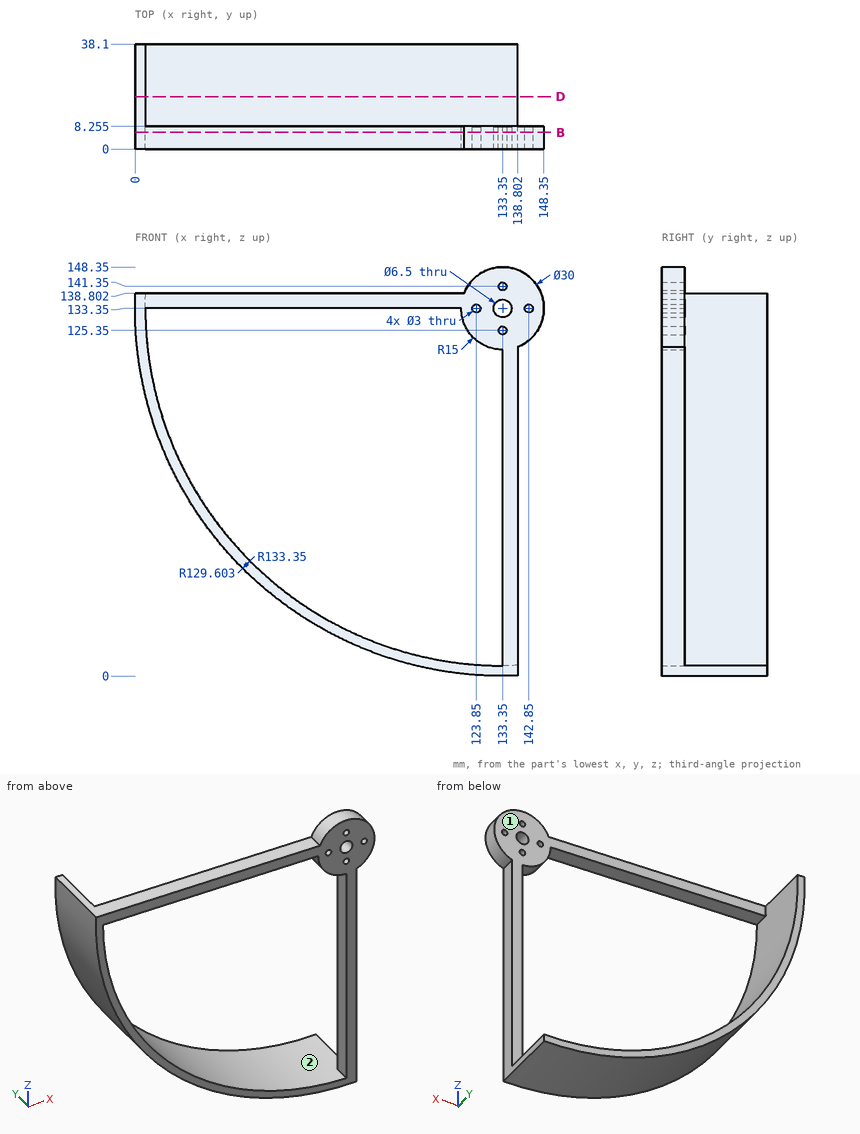
Here's the drawing with two shaded views (mm, measured from the low corner). I have some questions. Coordinates: 2 decimals unless noted, no trailing zeros. Write each loop counter-clockwise with the first axis right and the second up, starting at its lowest first coordinate (ties: lowest second). Pieces come first, ordered by that corner, then holes.
Item 1: I want a section at D-D on y = 19. Write out the boundary of the cut face in (x, z).
Item 2: If I drill on line 1 (Z direction, x = 123, y = 4) (1 decimal); line 2 (Z direction, x = 135, y = 6); line 3 (X direction, y = 5, z = 141.35), over which ranges is the centre line in solid material (lowest first)?
Item 3: I want a section at B-B on y = 6. Count the separate pieces of the cut face and the enclosed holes in it, and give its area (3 significant figures).
Item 4: Will these pins go through, and if not, where does the flat tip stop? pin 1 (19 mm diameter, centred on x = 66.5, y = 22, fed in from +Z); pin 2 (4 mm diameter, centred on x = 49, y = 6, fed in from -Z) (1 decimal); pin 3 (3 mm diameter, centred on y = 22, z = 68, fed in from -X); pin 4 (10.5 mm diameter, centred on x = 133.35, z = 133.35, fed in from -Y).
Item 5: If we mould it in two halves opening along Z, with no side actions, what happens to the marked faces 1 and 2? For each: +Z half, -Z half, draft (parallel to the pull), parting line (faces both ways), or undercut.
Findings below:
1. outline: (0.11, 138.8) arc R133.35 ccw to (138.8, 0.11) - (138.8, 3.86) arc R129.6 cw to (3.86, 138.8) - close
2. line 1: z = 0.4 to 4.2, 122.5 to 132.1, 134.6 to 144.2
2. line 2: z = 0.01 to 130.55, 136.15 to 148.26
2. line 3: x = 120.66 to 131.85, 134.85 to 146.04
3. separate pieces: 1
3. enclosed holes: 6
3. area: 2,710 mm2
4. pin 1: stops at z = 28.62
4. pin 2: stops at z = 28.5
4. pin 3: stops at x = 16.28
4. pin 4: stops at y = 0
5. face 1: draft
5. face 2: undercut
